from build123d import *

# Parameters (mm, degrees)
SKETCH1_W            = 96.0628
SKETCH1_H            = 90.3478
PCB_DEPTH            = 1.6256
SKETCH5_R            = 1.5875
PCB_HOLES_DEPTH      = 66.957101229
SKETCH6_W            = 57.15
SKETCH6_H            = 7.366
SKETCH6_H_2          = 9.398
PCB_EDGE_CONNS_DEPTH = 5.461


with BuildPart() as part:
    # Sketch1 → PCB (new body)
    with BuildSketch(Plane.XY):
        Rectangle(SKETCH1_W, SKETCH1_H)
    extrude(amount=PCB_DEPTH)

    # Sketch5 → PCB_Holes (cut, through all)
    with BuildSketch(Plane.XY.offset(1.6256)):
        with Locations((-42.7736, 36.83)):
            Circle(SKETCH5_R)
        with Locations((42.9514, 40.005)):
            Circle(SKETCH5_R)
        with Locations((42.9514, -40.005)):
            Circle(SKETCH5_R)
        with Locations((-42.7736, -36.83)):
            Circle(SKETCH5_R)
    extrude(amount=-PCB_HOLES_DEPTH, mode=Mode.SUBTRACT)

    # Sketch6 → PCB_Edge_Conns (add)
    with BuildSketch(Plane.XY.offset(1.6256)):
        with Locations((-6.7564, -46.0629)):
            Rectangle(SKETCH6_W, SKETCH6_H)
        with Locations((-6.7564, 45.0469)):
            Rectangle(SKETCH6_W, SKETCH6_H_2)
    extrude(amount=PCB_EDGE_CONNS_DEPTH)


solid = part.part
Input: part model. Units: mm. Frame: model coordinates. A direction names the side the tool comes from. Give positions to 0.01 mm unless a question says otherwise; leave off trailing zeros. Loops run counter-clockwise (first coordinate to the right, second up) from the corner with the lowest first, then second, coordinate; pieces in that order, holes last. Notation, with made-up numbers: M 16.5,19 L 47.5,19 A21 cw 47.5,26 Z; hole C 18,68.5 d4. An arc over 180 degrees is marked long. Use CSV: the item, a comma, the result in double quotes.
(1) Section A-A, the plane z = 3.25. Return loops of the section in (x, y).
Outcome:
outline,"M -35.33,-49.75 L 21.82,-49.75 L 21.82,-42.38 L -35.33,-42.38 Z; M -35.33,40.35 L 21.82,40.35 L 21.82,49.75 L -35.33,49.75 Z"
(2) Section B-B, the plane x = -10. Return loops of the section in (y, z).
Outcome:
outline,"M -49.75,1.63 L -45.17,1.63 L -45.17,0 L 45.17,0 L 45.17,1.63 L 49.75,1.63 L 49.75,7.09 L 40.35,7.09 L 40.35,1.63 L -42.38,1.63 L -42.38,7.09 L -49.75,7.09 Z"
(3) Pin query (flat end, axial travel): P1, Ø12, axis at x = 32.5, y = -24.5, coming from the +Z side; P2, Ø1.6, axis at y = 44, z = 4.5, coming from the -X side; P3, Ø1.4, axis at x = 0, y = 48, coming from the -Z side; P4, Ø5, axis at x = -16.5, y = -47, coming from the -Z side. Return the tip coordinate at first contact, or that it passes through.
Outcome:
P1,"stops at z = 1.63"
P2,"stops at x = -35.33"
P3,"stops at z = 1.63"
P4,"stops at z = 0"
(4) Section D-D, the plane y = 9. Return loops of the section in (x, z).
Outcome:
outline,"M -48.03,0 L 48.03,0 L 48.03,1.63 L -48.03,1.63 Z"
(5) Section C-C, the plane y = -36.83. Return loops of the section in (x, z).
Outcome:
outline,"M -48.03,0 L -44.36,0 L -44.36,1.63 L -48.03,1.63 Z; M -41.19,0 L 48.03,0 L 48.03,1.63 L -41.19,1.63 Z"
(6) Material intervals for L1, parallel to Y at x = -30, z = 4; L2, parallel to Z at x = -32, y = -13; L3, parallel to Y at x = 14, z = 0.75, sorted ascending. Write a range as [from, to].
Outcome:
L1,"y = [-49.75, -42.38], [40.35, 49.75]"
L2,"z = [0, 1.63]"
L3,"y = [-45.17, 45.17]"
(7) Pull-direction query (X, two-part tool) for faces 6 (the face through (-35.331, 45, 4)), 7 (the face through (43.684, 38.597, 0.824)), 8 (the face through (-7, -46, 7.087)); classes: pulls with the +X half, pulls with the -X half, needs draft (parallel to the pull), parting line crosses it, or undercut.
Outcome:
face 6,"pulls with the -X half"
face 7,"undercut"
face 8,"needs draft"
(8) Set-up query: faces 1 (the face through (-7, 47, 1.626)), 2 (the face through (-7, -42.38, 4)), 3 (the face through (-35.331, -46, 4)), 4 (the face through (-7, -47, 1.626)), 5 (the face through (21.819, -46, 4)). Return all of +Z, -Z, +X, -X, +Y, -Y with unobstructed straight access to the full face (end or side cutting, diameter ignored); none if empty.
Outcome:
face 1,"-Z, +X, -X, +Y"
face 2,"+Z, +X, -X"
face 3,"+Z, -X, +Y, -Y"
face 4,"-Z, +X, -X, -Y"
face 5,"+Z, +X, +Y, -Y"
